```python
from build123d import *

# Parameters (mm, degrees)
BOSS_EXTRUDE1_DEPTH = 223.6
SKETCH2_R           = 4
SKETCH2_R_2         = 6
CUT_EXTRUDE1_DEPTH  = 226.617397379


with BuildPart() as part:
    # Sketch1 → Boss-Extrude1 (new, symmetric)
    with BuildSketch(Plane.XY):
        Polygon((2.5, 2.5), (0, 2.5), (0, 0), (30, 0), (30, 2.5), align=None)
    extrude(amount=BOSS_EXTRUDE1_DEPTH, both=True)

    # Sketch2 → Cut-Extrude1 (cut, through all)
    with BuildSketch(Plane(origin=(0, 2.5, 0), x_dir=(1, 0, 0), z_dir=(0, 1, 0))):
        with Locations(Location((12.5, 211.1, 0), (0, 0, 180))):
            Circle(SKETCH2_R)
        with Locations((12.5, -211.1)):
            Circle(SKETCH2_R)
        with Locations(Location((15, -100, 0), (0, 0, 180))):
            Circle(SKETCH2_R_2)
        with Locations((15, 100)):
            Circle(SKETCH2_R_2)
        with Locations(Location((15, 0, 0), (0, 0, 180))):
            Circle(SKETCH2_R_2)
    extrude(amount=-CUT_EXTRUDE1_DEPTH, mode=Mode.SUBTRACT)


solid = part.part
```
The listing builds one solid part. Answer for the finished solid, in the listing's coordinates (mm). Give positions to 0.01 mm unless a question says otherwise; leave off trailing zeros. Write each loop counter-clockwise with the first axis right and the second up, starting at its lowest first coordinate (ties: lowest second). Pieces come first, ordered by that corner, then holes. Notation, with made-up numbers: (86, 6) - (142, 6) arc R31 cw to (142, 31) - close; hole circle Ø3 at (33, 34). An arc over 180 degrees is marked (long way). Use one line per item in the form item = value. Start each with the question number.
1) Find section C-C on z = 100. Determine the outline of the cut face in (x, y).
2) Find section B-B on y = 1.65. Determine the outline of the cut face in (x, z), plus the area to 3 significant figures.
3) The mould has two halves that part along Z. Classify faces 1 (the face through (11.979, 1.268, 207.134)), 2 (the face through (22, 2.5, 3)): pulls with the +Z half, pulls with the -Z half, needs draft (parallel to the pull), parting line crosses it, or undercut.
4) Consider line 1 along X through (y, z) = (0.5, -100); line 2 along Z through (x, y) = (20, 2); line 3 along Z through (x, y) = (15, 0.65). Determine where each line is inside the solid, lowest interval first. Write a range as from..to.
5) Find section A-A on z = -211.1. Determine the outline of the cut face in (x, y).
Geometry results:
q1.outline = (0, 0) - (9, 0) - (9, 2.5) - (0, 2.5) - close; (21, 0) - (30, 0) - (30, 2.5) - (21, 2.5) - close
q2.outline = (0, -223.6) - (30, -223.6) - (30, 223.6) - (0, 223.6) - close; hole circle Ø8 at (12.5, -211.1); hole circle Ø8 at (12.5, 211.1); hole circle Ø12 at (15, -100); hole circle Ø12 at (15, 0); hole circle Ø12 at (15, 100)
q2.area = 13,000 mm2
q3.face_1 = undercut
q3.face_2 = needs draft
q4.line_1 = 0..9, 21..30
q4.line_2 = -223.6..-103.32, -96.68..-3.32, 3.32..96.68, 103.32..223.6
q4.line_3 = -223.6..-214.22, -207.98..-106, -94..-6, 6..94, 106..207.98, 214.22..223.6
q5.outline = (0, 0) - (8.5, 0) - (8.5, 2.5) - (0, 2.5) - close; (16.5, 0) - (30, 0) - (30, 2.5) - (16.5, 2.5) - close
